Could you check a few things on this drawing? It's one solid part, dimensions in mm from its lowest x, y, z. A direction names the side the tool comes from. Give positions to 0.01 mm unless a question says otherwise; leave off trailing zeros. Loops run counter-clockwise (first coordinate to the right, second up) from the corner with the lowest first, then second, coordinate; pieces in that order, holes last.
1. For the marked faces 1, 2, 3, 4 and 5, which set-ups out of +Z, -Z, +X, -X, +Y, -Y let a thin tool reach every point of the face, with its end or its side?
2. Imagine slicing it at C-C (x = 11). List the corners of the cut face in (y, z) for me.
3. I need wall thicknesses on line 1 along X through (y, z) = (18, 2.75) (1 decimal); line 2 along Y through (x, z) = (9, 1.25); line 3 along X through (y, z) = (17, 8.25) (1 decimal). Which ranges of each line are inside material? Lowest first, please.
4. Imagine slicing it at D-D (y = 11.5). List the corners of the cut face in (x, z) for me, plus the area to 4 significant figures.
5. Imagine slicing it at A-A (z = 2.54). List the corners of the cut face in (x, y) for me (3 decimals).
6. For P1, Ø6, axis at y = 5.5, z = 6.5, coming from the -X side; P2, Ø2.5, axis at x = 29.845, z = 9.144, coming from the +Y side; P3, Ø6, axis at x = 18, z = 6, coming from the +Y side; P4, Ø1, axis at x = 16, z = 10, coming from the -Y side, each with a flat end and sliding along its axis, tell me the tip position at first contact or that it passes through.
7. Imagine slicing it at B-B (x = 2.54). List the corners of the cut face in (y, z) for me, plus the area to 3 significant figures.
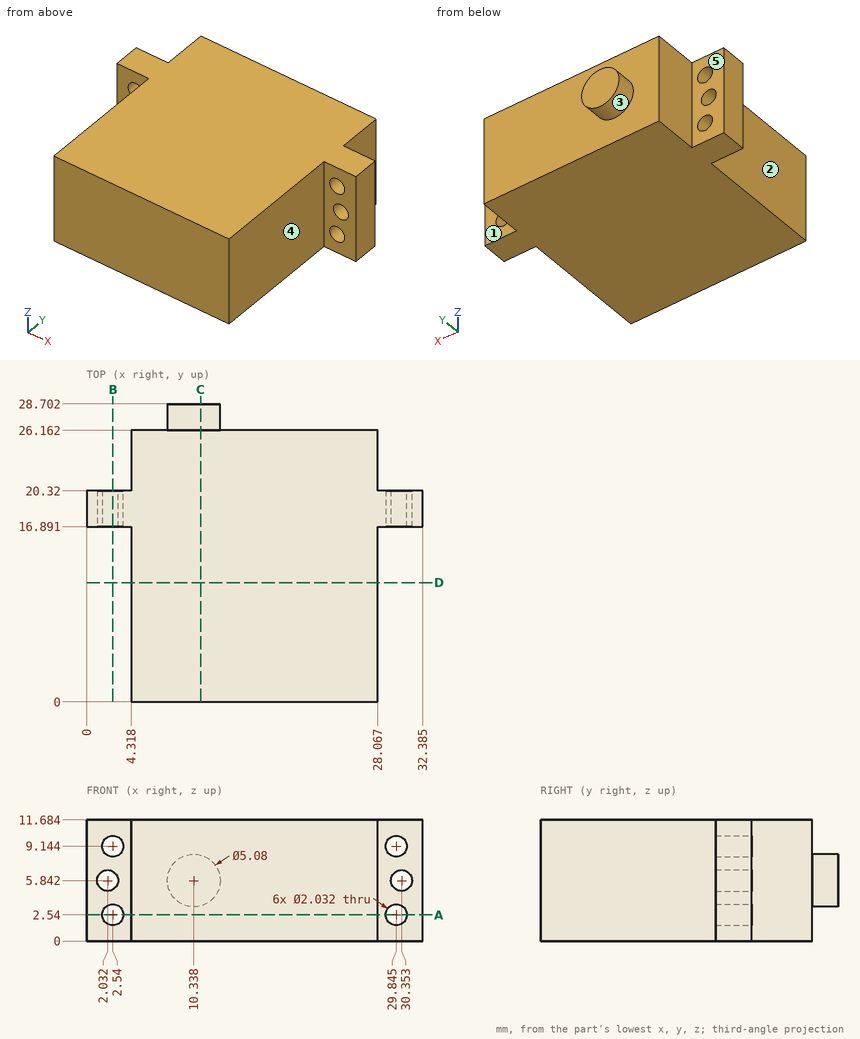
Derived:
1. face 1: +Z, -Z, +X, +Y
1. face 2: +Z, -Z, -X, -Y
1. face 3: +Y
1. face 4: +Z, -Z, +X, -Y
1. face 5: +Z, -Z, -X, +Y
2. outline: (0, 0) - (26.16, 0) - (26.16, 3.39) - (28.7, 3.39) - (28.7, 8.29) - (26.16, 8.29) - (26.16, 11.68) - (0, 11.68) - close
3. line 1: x = 0 to 1.5, 3.5 to 28.9, 30.8 to 32.4
3. line 2: y = 0 to 26.16
3. line 3: x = 0 to 2.1, 3 to 29.4, 30.3 to 32.4
4. outline: (4.32, 0) - (28.07, 0) - (28.07, 11.68) - (4.32, 11.68) - close
4. area: 277.5 mm2
5. outline: (0, 16.891) - (1.524, 16.891) - (1.524, 20.32) - (0, 20.32) - close; (3.556, 16.891) - (4.318, 16.891) - (4.318, 0) - (28.067, 0) - (28.067, 16.891) - (28.829, 16.891) - (28.829, 20.32) - (28.067, 20.32) - (28.067, 26.162) - (4.318, 26.162) - (4.318, 20.32) - (3.556, 20.32) - close; (30.861, 16.891) - (32.385, 16.891) - (32.385, 20.32) - (30.861, 20.32) - close
6. P1: stops at x = 4.32
6. P2: stops at y = 20.32
6. P3: stops at y = 26.16
6. P4: stops at y = 0
7. outline: (16.89, 0) - (20.32, 0) - (20.32, 1.52) - (16.89, 1.52) - close; (16.89, 3.56) - (20.32, 3.56) - (20.32, 4.96) - (16.89, 4.96) - close; (16.89, 6.72) - (20.32, 6.72) - (20.32, 8.13) - (16.89, 8.13) - close; (16.89, 10.16) - (20.32, 10.16) - (20.32, 11.68) - (16.89, 11.68) - close
7. area: 20.1 mm2
